Check sheet for the modelled part. Datum: model origin and axes. Units: mm. A direction names the side the tool comes from. Round coordinates to 2 decimals unless told otherwise and drop trailing zeros. Write each loop counter-clockwise with the first axis right and the second up, starting at its lowest first coordinate (ties: lowest second). Pieces come first, ordered by that corner, then holes. Notation, with made-up numbers: (-20.5, 31) -> (-13.5, 31) arc R20 cw to (-13.5, 66) -> close; hole circle Ø3 at (27, 54). An arc over 180 degrees is marked (long way). Put each result on its own line as item: value. Start each with the question number.
from build123d import *

# Parameters (mm, degrees)
EXTRUDE_1_DEPTH        = 20
FILLET_2_R             = 10
EXTRUDE_2_DEPTH        = 20
SKETCH_6_R             = 5
CUT_EXTRUDE_1_DEPTH    = 20
FILLET_2_OF_MIRROR_3_R = 10
SKETCH_8_W             = 30
SKETCH_8_H             = 20
CUT_EXTRUDE_2_DEPTH    = 215.941852602


with BuildPart() as part:
    # 草图4 → 凸台-拉伸1 (new body)
    with BuildSketch(Plane.XY):
        Polygon((0, 0), (-30, 0), (-30, 90), (30, 170), (70, 170), (70, 150), (45, 150), (0, 90), align=None)
    extrude_1 = extrude(amount=EXTRUDE_1_DEPTH)

    # 圆角2
    fillet_2_edges = [part.edges().sort_by_distance(p)[0] for p in [
        (70, 160, 0),
        (70, 170, 10),
        (70, 150, 10),
        (70, 160, 20),
    ]]
    fillet(fillet_2_edges, radius=FILLET_2_R - 0.0001)  # a hair under: the kernel refuses the full size

    # 草图5 → 凸台-拉伸2 (add)
    with BuildSketch(Plane(origin=(0, 0, 0), x_dir=(-1, 0, 0), z_dir=(0, 0, -1))):
        with BuildLine():
            ThreePointArc((7.928932188, 22.071067812), (5, 15), (7.928932188, 7.928932188))
            Line((7.928932188, 7.928932188), (15, 15))
            Line((15, 15), (7.928932188, 22.071067812))
        make_face()
        with BuildLine():
            Line((15, 15), (7.928932188, 7.928932188))
            ThreePointArc((7.928932188, 7.928932188), (15, 5), (22.071067812, 7.928932188))
            Line((22.071067812, 7.928932188), (15, 15))
        make_face()
        with BuildLine():
            Line((15, 15), (22.071067812, 7.928932188))
            ThreePointArc((22.071067812, 7.928932188), (24.238795325, 11.173165676), (25, 15))
            ThreePointArc((25, 15), (24.238795325, 18.826834324), (22.071067812, 22.071067812))
            Line((22.071067812, 22.071067812), (15, 15))
        make_face()
        with BuildLine():
            ThreePointArc((22.071067812, 22.071067812), (15, 25), (7.928932188, 22.071067812))
            Line((7.928932188, 22.071067812), (15, 15))
            Line((15, 15), (22.071067812, 22.071067812))
        make_face()
    extrude_2 = extrude(amount=EXTRUDE_2_DEPTH)

    # 草图6 → 切除-拉伸1 (cut)
    with BuildSketch(Plane.XY.offset(20)):
        with Locations((4, 112)):
            Circle(SKETCH_6_R)
    cut_extrude_1 = extrude(amount=-CUT_EXTRUDE_1_DEPTH, mode=Mode.SUBTRACT)

    # 镜向3: 凸台-拉伸1, 凸台-拉伸2, 切除-拉伸1 across plane
    add(extrude_1.mirror(Plane(origin=(-30, 0, 20), x_dir=(0, 0, 1), z_dir=(1, 0, 0))))
    add(extrude_2.mirror(Plane(origin=(-30, 0, 20), x_dir=(0, 0, 1), z_dir=(1, 0, 0))))
    add(cut_extrude_1.mirror(Plane(origin=(-30, 0, 20), x_dir=(0, 0, 1), z_dir=(1, 0, 0))), mode=Mode.SUBTRACT)

    # 圆角2 of 镜向3
    fillet_2_of_mirror_3_edges = [part.edges().sort_by_distance(p)[0] for p in [
        (-130, 160, 0),
        (-130, 170, 10),
        (-130, 150, 10),
        (-130, 160, 20),
    ]]
    fillet(fillet_2_of_mirror_3_edges, radius=FILLET_2_OF_MIRROR_3_R - 0.0001)  # a hair under: the kernel refuses the full size

    # 草图8 → 切除-拉伸2 (cut, through all)
    with BuildSketch(Plane.XZ):
        Polygon((88.976151269, 20), (0, 20), (0, 0), (-30, 0), (-30, -22.976425092), (88.976151269, -22.976425092), align=None)
        with Locations((-15, 10)):
            Rectangle(SKETCH_8_W, SKETCH_8_H)
    extrude(amount=-CUT_EXTRUDE_2_DEPTH, mode=Mode.SUBTRACT)


solid = part.part
1. Draft check along Y on faces 3 (the cylindrical face through (-62.92, 107.12, 10.14)), 4 (the flat face through (-45, 15, -20)), 5 (the flat face through (-59.58, 129.44, 9.86)). Enter one of: released by +Y, released by -Y, zero draft, split by the parting line, or undercut.
2. Section check C-C, the plane x = -64. Enter the section's corners in (y, z), then the cut area to 3 significant figures.
3. Section check A-A, the plane y = 112. Enter the section's corners in (x, z), then the cut area to 3 significant figures.
4. Section check D-D, the plane x = -41.5. Enter the section's corners in (y, z), then the cut area to 3 significant figures.
5. Gauge pin test, flat ends, axial feed: P1, Ø8, axis at x = -64, y = 112, coming from the -Z side; P2, Ø6, axis at y = 62, z = 11, coming from the -X side; P3, Ø12, axis at x = -60.5, z = -2.5, coming from the +Y side; P4, Ø6, axis at x = -66.5, y = 111.5, coming from the -Z side. Record the tip position at first contact, or that the pin passes through.
6. Material ranges on L1, parallel to Z at x = -56.5, y = 18.5; L2, parallel to Y at x = -64, z = 15.5; L3, parallel to X at y = 17.5, z = 14, recorded low to high. Write a range as [from, to].
7. Section check B-B, the plane z = 13.5. Enter the section's corners in (x, y).
8. Access from +Z, -Z, +X, -X, +Y, -Y to the whole of each face (thin tool, end or side, straight path). Record for faces 1 (the flat face through (-113, 150, 10)), 2 (the cylindrical face through (-126, 160, 18)).
Reply:
1. face 3: undercut
1. face 4: zero draft
1. face 5: released by +Y
2. outline: (95.33, 0) -> (107, 0) -> (107, 20) -> (95.33, 20) -> close; (117, 0) -> (135.33, 0) -> (135.33, 20) -> (117, 20) -> close
2. area: 600 mm2
3. outline: (-76.5, 0) -> (-69, 0) -> (-69, 20) -> (-76.5, 20) -> close; (-59, 0) -> (-46.5, 0) -> (-46.5, 20) -> (-59, 20) -> close
3. area: 400 mm2
4. outline: (0, 0) -> (5.63, 0) -> (5.63, -20) -> (24.37, -20) -> (24.37, 0) -> (105.33, 0) -> (105.33, 20) -> (0, 20) -> close
4. area: 2,480 mm2
5. P1: passes through
5. P2: stops at x = -60
5. P3: stops at y = 137.94
5. P4: stops at z = 0
6. L1: z = [0, 20]
6. L2: y = [95.33, 107], [117, 135.33]
6. L3: x = [-60, -30]
7. outline: (-129.37, 156.5) arc R10 ccw to (-120, 150) -> (-105, 150) -> (-60, 90) -> (-60, 0) -> (-30, 0) -> (-30, 90) -> (-90, 170) -> (-120, 170) arc R10 ccw to (-129.37, 163.5) -> close; hole circle Ø10 at (-64, 112)
8. face 1: +Z, -Z, -X, -Y
8. face 2: +Z, -X, +Y, -Y
